```python
from build123d import *

# Parameters (mm, degrees)
EXTRUDE_1_DEPTH     = 2.4
SKETCH_2_R          = 1.5
CUT_EXTRUDE_1_DEPTH = 10
FILLET_1_R          = 0.5
EXTRUDE_START       = 1.1
SKETCH_3_R          = 2.7
SKETCH_3_R_2        = 1.5
EXTRUDE_2_DEPTH     = 1.1
FILLET_2_R          = 0.5


with BuildPart() as part:
    # 草图1 → 凸台-拉伸1 (new body)
    with BuildSketch(Plane(origin=(0, 0, 0), x_dir=(1, 0, 0), z_dir=(0, 1, 0))):
        Polygon((0, 3.117691454), (-2.7, 1.558845727), (-2.7, -1.558845727), (0, -3.117691454), (2.7, -1.558845727), (2.7, 1.558845727), align=None)
    extrude(amount=EXTRUDE_1_DEPTH)

    # 草图2 → 切除-拉伸1 (cut)
    with BuildSketch(Plane(origin=(0, 2.4, 0), x_dir=(1, 0, 0), z_dir=(0, 1, 0))):
        with Locations(Location((0, 0, 0), (0, 0, 270))):
            Circle(SKETCH_2_R)
    extrude(amount=-CUT_EXTRUDE_1_DEPTH, mode=Mode.SUBTRACT)

    # 圆角1
    fillet_1_edges = [part.edges().sort_by_distance(p)[0] for p in [
        (-2.7, 2.4, 0),
        (-1.35, 2.4, 2.33826859),
        (1.35, 2.4, 2.33826859),
        (2.7, 2.4, 0),
        (1.35, 2.4, -2.33826859),
        (2.7, 0, 0),
        (1.35, 0, 2.33826859),
        (-1.35, 0, 2.33826859),
        (-2.7, 0, 0),
        (-1.35, 0, -2.33826859),
        (1.35, 0, -2.33826859),
        (-1.35, 2.4, -2.33826859),
    ]]
    fillet(fillet_1_edges, radius=FILLET_1_R)

    # 草图3 → 凸台-拉伸2 (add)
    with BuildSketch(Plane(origin=(0, 2.4, 0), x_dir=(1, 0, 0), z_dir=(0, 1, 0)).offset(EXTRUDE_START)):
        with Locations(Location((0, 0, 0), (0, 0, 270))):
            Circle(SKETCH_3_R)
        with Locations(Location((0, 0, 0), (0, 0, 270))):
            Circle(SKETCH_3_R_2, mode=Mode.SUBTRACT)
    extrude(amount=-EXTRUDE_2_DEPTH)

    # 圆角2
    fillet_2_edges = [part.edges().sort_by_distance(p)[0] for p in [
        (0, 3.5, -2.7),
        (0, 3.5, -1.5),
    ]]
    fillet(fillet_2_edges, radius=FILLET_2_R)


solid = part.part
```
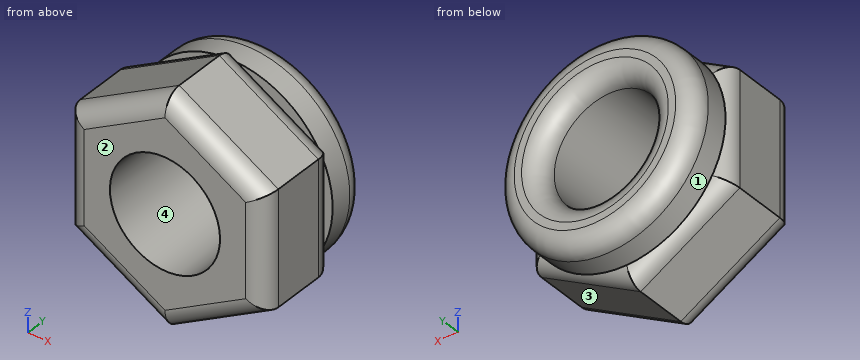
Here's how the part is built. I have some questions about the finished solid (model axes, mm). Face numbers are marked on the shaded views. Give positions to 0.01 mm unless a question says otherwise; leave off trailing zeros. Order: outer loops, then holes, each group sorted by start corner. A loop starts at its lowest first (then second) coordinate and runs counter-clockwise, first axis right, second up. Notation, with made-up numbers: (-31.5, -32.5) - (15.5, -32.5) arc R30 ccw to (15.5, -8.5) - close; hole circle Ø8 at (0, 31.25). An arc over 180 degrees is marked (long way). Answer as a JSON object with one key per item and string values. Group by question number.
Item 1: If we section it at C-C on y = 2.2: Please give me the cut outline in (x, z), and give its area (3 significant figures).
Item 2: For P1, Ø1, axis at x = 1, y = 1, coming from the +Z side, with a flat end and sliding along its axis, tell me the tip position at first contact or that it passes through.
Item 3: If we section it at B-B on y = 1.7: Please give me the cut outline in (x, z).
Item 4: Please list where these lines run through material, in increasing order: probe 1 along X at (y, z) = (1.7, 0); probe 2 along X at (y, z) = (0.7, -1); probe 3 along Z at (x, y) = (-1.15, 3.25).
Item 5: If we section it at A-A on z = 0: Please give me the cut outline in (x, y), and give its area (3 significant figures).
Item 6: If we mould it in two halves opening along Z, with no side actions, what happens to the marked faces 1, 2, 3 and 4? For each: pulls with the +Z half, pulls with the -Z half, needs draft (parallel to the pull), parting line crosses it, or undercut.
Result set:
{
 "1": {"outline": "(-2.6, -1.5) - (0, -3) - (2.6, -1.5) - (2.6, 1.5) - (0, 3) - (-2.6, 1.5) - close; hole circle Ø3 at (0, 0)", "area": "16.3 mm²"},
 "2": {"P1": "z = 2.83"},
 "3": {"outline": "(-2.7, -1.56) - (0, -3.12) - (2.7, -1.56) - (2.7, 1.56) - (0, 3.12) - (-2.7, 1.56) - close; hole circle Ø3 at (0, 0)"},
 "4": {"probe 1": "-2.7 to -1.5, 1.5 to 2.7", "probe 2": "-2.7 to -1.12, 1.12 to 2.7", "probe 3": "-2.37 to -1.06, 1.06 to 2.37"},
 "5": {"outline": "(-2.7, 0.5) arc R0.5 ccw to (-2.2, 0) - (-1.5, 0) - (-1.5, 3) arc R0.5 ccw to (-2, 3.5) - (-2.2, 3.5) arc R0.5 ccw to (-2.7, 3) - (-2.7, 2.4) - (-2.2, 2.4) arc R0.5 ccw to (-2.7, 1.9) - close; (1.5, 0) - (2.2, 0) arc R0.5 ccw to (2.7, 0.5) - (2.7, 1.9) arc R0.5 ccw to (2.2, 2.4) - (2.7, 2.4) - (2.7, 3) arc R0.5 ccw to (2.2, 3.5) - (2, 3.5) arc R0.5 ccw to (1.5, 3) - close", "area": "7.97 mm²"},
 "6": {"face 1": "parting line crosses it", "face 2": "needs draft", "face 3": "pulls with the -Z half", "face 4": "undercut"}
}
